Work out the finished part from the listing and answer in its coordinate system (mm). A direction names the side the tool comes from. Round coordinates to 2 decimals unless told otherwise and drop trailing zeros. Loops run counter-clockwise (first coordinate to the right, second up) from the corner with the lowest first, then second, coordinate; pieces in that order, holes last. Notation, with made-up numbers: (42, 62) - (97, 62) arc R10 ccw to (97, 78) - close; hole circle Ø6 at (83, -12.75). An arc over 180 degrees is marked (long way). Return JSON: item names as keys, results as strings.
from build123d import *

# Parameters (mm, degrees)
BOSS_EXTRUDE1_DEPTH = 15
SKETCH2_W           = 15
SKETCH2_H           = 10
BOSS_EXTRUDE2_DEPTH = 19.8
SKETCH3_W           = 5
SKETCH3_H           = 15
CUT_EXTRUDE1_DEPTH  = 40
CUT_EXTRUDE2_REACH  = 89.134
SKETCH4_R           = 1.7
LPATTERN1_COUNT     = 2
LPATTERN1_PITCH     = 14
CUT_EXTRUDE3_DEPTH  = 2.5
CUT_EXTRUDE4_DEPTH  = 15
FILLET1_R           = 7.5


with BuildPart() as part:
    # Sketch1 → Boss-Extrude1 (new body)
    with BuildSketch(Plane(origin=(0, 0, 0), x_dir=(1, 0, 0), z_dir=(0, 1, 0))):
        Polygon((-27.5, 0), (27.5, 0), (27.5, 85), (14.5, 85), (14.5, 18), (7.7, 18), (7.7, 10), (-7.7, 10), (-7.7, 18), (-14.5, 18), (-14.5, 85), (-27.5, 85), align=None)
    extrude(amount=BOSS_EXTRUDE1_DEPTH)

    # Sketch2 → Boss-Extrude2 (add)
    with BuildSketch(Plane(origin=(0, 15, 0), x_dir=(1, 0, 0), z_dir=(0, 1, 0))):
        with Locations((0, 5)):
            Rectangle(SKETCH2_W, SKETCH2_H)
    extrude(amount=BOSS_EXTRUDE2_DEPTH)

    # Sketch3 → Cut-Extrude1 (cut)
    with BuildSketch(Plane(origin=(0, 0, -85), x_dir=(-1, 0, 0), z_dir=(0, 0, -1))):
        with Locations((22, 7.5)):
            Rectangle(SKETCH3_W, SKETCH3_H)
        with Locations((-22, 7.5)):
            Rectangle(SKETCH3_W, SKETCH3_H)
    extrude(amount=-CUT_EXTRUDE1_DEPTH, mode=Mode.SUBTRACT)

    # Sketch4 → Cut-Extrude2 (cut, up to next)
    with BuildSketch(Plane(origin=(0, 0, -10), x_dir=(-1, 0, 0), z_dir=(0, 0, -1)), mode=Mode.PRIVATE) as cut_extrude2_sk1:
        with Locations((-3.5, 28)):
            Circle(SKETCH4_R)
    cut_extrude2_tool1 = extrude(cut_extrude2_sk1.sketch, amount=-CUT_EXTRUDE2_REACH, mode=Mode.PRIVATE) & part.part
    # Sketch4 → Cut-Extrude2 (cut, up to next)
    with BuildSketch(Plane(origin=(0, 0, -10), x_dir=(-1, 0, 0), z_dir=(0, 0, -1)), mode=Mode.PRIVATE) as cut_extrude2_sk2:
        with Locations((3.5, 21)):
            Circle(SKETCH4_R)
    cut_extrude2_tool2 = extrude(cut_extrude2_sk2.sketch, amount=-CUT_EXTRUDE2_REACH, mode=Mode.PRIVATE) & part.part
    cut_extrude2_1 = cut_extrude2_tool1.solids().sort_by_distance((3.5, 28, -10))[0]
    add(cut_extrude2_1, mode=Mode.SUBTRACT)
    cut_extrude2_2 = cut_extrude2_tool2.solids().sort_by_distance((-3.5, 21, -10))[0]
    add(cut_extrude2_2, mode=Mode.SUBTRACT)
    cut_extrude2 = cut_extrude2_1 + cut_extrude2_2  # Cut-Extrude2 as one shape, for the pattern or mirror that repeats it

    # LPattern1: Cut-Extrude2 ×2
    with Locations(*[(0, -i * LPATTERN1_PITCH, 0) for i in range(1, LPATTERN1_COUNT)]):
        add(cut_extrude2, mode=Mode.SUBTRACT)

    # Sketch5 → Cut-Extrude3 (cut)
    with BuildSketch(Plane.ZY.offset(-14.5)):
        Polygon((-79.25, 10.531088913), (-45.75, 10.531088913), (-44, 7.5), (-45.75, 4.468911087), (-79.25, 4.468911087), (-81, 7.5), align=None)
    cut_extrude3 = extrude(amount=-CUT_EXTRUDE3_DEPTH, mode=Mode.SUBTRACT)

    # Sketch6 → Cut-Extrude4 (cut)
    with BuildSketch(Plane.ZY.offset(-17)):
        with BuildLine():
            Line((-77.5, 9.088089066), (-47.5, 9.2))
            ThreePointArc((-47.5, 9.2), (-45.811011578, 7.693178963), (-47.116144669, 5.843903661))
            Line((-47.116144669, 5.843903661), (-77.503554355, 5.911914911))
            ThreePointArc((-77.503554355, 5.911914911), (-79.088088072, 7.501777179), (-77.5, 9.088089066))
        make_face()
    cut_extrude4 = extrude(amount=-CUT_EXTRUDE4_DEPTH, mode=Mode.SUBTRACT)

    # Mirror1: Cut-Extrude3, Cut-Extrude4 across plane
    add(cut_extrude3.mirror(Plane(origin=(0, 0, 0), x_dir=(0, 0, 1), z_dir=(1, 0, 0))), mode=Mode.SUBTRACT)
    add(cut_extrude4.mirror(Plane(origin=(0, 0, 0), x_dir=(0, 0, 1), z_dir=(1, 0, 0))), mode=Mode.SUBTRACT)

    # Fillet1
    fillet1_edges = [part.edges().sort_by_distance(p)[0] for p in [
        (26, 15, -85),
        (17, 15, -85),
        (-17, 15, -85),
        (-26, 15, -85),
        (26, 0, -85),
        (17, 0, -85),
        (-17, 0, -85),
        (-26, 0, -85),
    ]]
    fillet(fillet1_edges, radius=FILLET1_R - 0.0001)  # a hair under: the kernel refuses the full size


solid = part.part
1) Flat-ended cylindrical pins translate along their axes: pin 1 (10 mm diameter, centred on y = 26.5, z = -10.5, fed in from +X); pin 2 (1.5 mm diameter, centred on x = -22, y = 5, fed in from -Z); pin 3 (4 mm diameter, centred on x = 3.5, y = 14, fed in from -Z). Find the tip coordinate at first contact, or state that the pin passes through.
Verdict:
{"pin 1": "stops at x = 7.5", "pin 2": "stops at z = -45", "pin 3": "stops at z = -10"}
2) Section C-C (z = -52.5) is taken. Count the separate pieces of the cut face and the enclosed holes in it, and give its area (3 significant figures).
Verdict:
{"separate pieces": "8", "enclosed holes": "0", "area": "173 mm2"}
3) Section D-D (y = 14) is taken. Give the vertices of the cut face in (x, z).
Verdict:
{"outline": "(-27.5, -81.24) - (-24.5, -81.24) - (-24.5, -45) - (-19.5, -45) - (-19.5, -81.24) - (-14.5, -81.24) - (-14.5, -18) - (-7.7, -18) - (-7.7, -10) - (1.8, -10) - (1.8, 0) - (-27.5, 0) - close; (5.2, -10) - (7.7, -10) - (7.7, -18) - (14.5, -18) - (14.5, -81.24) - (19.5, -81.24) - (19.5, -45) - (24.5, -45) - (24.5, -81.24) - (27.5, -81.24) - (27.5, 0) - (5.2, 0) - close"}
4) Find the intervals of material crossed by L1, parallel to Y at x = 3.5, z = -5; L2, parallel to Y at x = -3.5, z = -5; L3, parallel to X at y = 11, z = -48, in increasing order.
Verdict:
{"L1": "y = 0 to 12.3, 15.7 to 26.3, 29.7 to 34.8", "L2": "y = 0 to 5.3, 8.7 to 19.3, 22.7 to 34.8", "L3": "x = -27.5 to -24.5, -19.5 to -14.5, 14.5 to 19.5, 24.5 to 27.5"}
5) A tool of negligible diameter and unlimited length cuts with its end or side. For faces 5 (the flat face through (-24.5, 5.7, -65.3)), 6 (the cylindrical face through (-18.232, 7.467, -79.088)), 7 (the flat face through (17, 5.5, -62.2)), from which of +Z, -Z, +X, -X, +Y, -Y can it reach the whole face along a straight path? Write none if from no direction.
Verdict:
{"face 5": "-Z, +Y, -Y", "face 6": "+X, -X", "face 7": "none"}
6) Section B-B (y = 28) is taken. Give the vertices of the cut face in (x, z), and give its area (3 significant figures).
Verdict:
{"outline": "(-7.5, -10) - (1.8, -10) - (1.8, 0) - (-7.5, 0) - close; (5.2, -10) - (7.5, -10) - (7.5, 0) - (5.2, 0) - close", "area": "116 mm2"}
7) Section A-A (x = -3.5) is taken. Give the vertices of the cut face in (y, z).
Verdict:
{"outline": "(0, -10) - (5.3, -10) - (5.3, 0) - (0, 0) - close; (8.7, -10) - (19.3, -10) - (19.3, 0) - (8.7, 0) - close; (22.7, -10) - (34.8, -10) - (34.8, 0) - (22.7, 0) - close"}
8) Determine the mould class of faces 1 (the flat face through (-16, 4.469, -62)), 2 (the flat face through (7.5, 25, -5)), 3 (the cylindrical face through (18.232, 7.467, -79.088)), 4 (the flat face through (-15.73, 6.01, -44.86)) for opening direction X: pulls with the +X half, pulls with the -X half, needs draft (parallel to the pull), parting line crosses it, or undercut.
Verdict:
{"face 1": "undercut", "face 2": "pulls with the +X half", "face 3": "needs draft", "face 4": "undercut"}
